Read the model definition and answer for the solid it produces. Units are mm, in the model's axes. A direction names the side the tool comes from. Give positions to 0.01 mm unless a question says otherwise; leave off trailing zeros. Write each loop counter-clockwise with the first axis right and the second up, starting at its lowest first coordinate (ties: lowest second). Pieces come first, ordered by that corner, then holes. Notation, with made-up numbers: M 40,19.25 L 64,19.25 A10 ccw 64,31.25 Z; hole C 73,48 d3. An arc over 180 degrees is marked long. Answer as CSV lines item,"result". Start each with the question number.
```python
from build123d import *

# Parameters (mm, degrees)
EXTRUDE_THIN1_DEPTH       = 100
BOSS_EXTRUDE1_START       = -10
BOSS_EXTRUDE1_DEPTH       = 10
SKETCH3_R                 = 2.25
BOSS_EXTRUDE2_DEPTH       = 5
BOSS_EXTRUDE3_DEPTH       = 10
SKETCH5_R                 = 2.25
CUT_EXTRUDE1_DEPTH        = 6
BOSS_EXTRUDE4_REACH       = 121.416
BOSS_EXTRUDE4_END_RADIUS  = 39
SKETCH10_W                = 20
SKETCH10_H                = 20
BOSS_EXTRUDE5_START       = -19.757252304
BOSS_EXTRUDE5_OUTLINE_W   = 20
BOSS_EXTRUDE5_OUTLINE_H   = 20
BOSS_EXTRUDE5_DEPTH       = 19.757252304
BOSS_EXTRUDE5_START_2     = 71.178890271
BOSS_EXTRUDE5_2_OUTLINE_W = 23
BOSS_EXTRUDE5_2_OUTLINE_H = 23
BOSS_EXTRUDE5_2_DEPTH     = 1.821109729
BOSS_EXTRUDE6_DEPTH       = 20
SKETCH12_R                = 2.5
CUT_EXTRUDE2_DEPTH        = 20


with BuildPart() as part:
    # Sketch1 → Extrude-Thin1 (new body)
    with BuildSketch(Plane.XY):
        with BuildLine():
            ThreePointArc((-35, 0), (0, -35), (35, 0))
            Line((35, 0), (39, 0))
            ThreePointArc((39, 0), (0, -39), (-39, 0))
            Line((-39, 0), (-35, 0))
        make_face()
    extrude(amount=EXTRUDE_THIN1_DEPTH)

    # Sketch2 → Boss-Extrude1 (add)
    with BuildSketch(Plane.XY.offset(100).offset(BOSS_EXTRUDE1_START)):
        with BuildLine():
            Line((0, -39), (0, -35))
            Line((0, -35), (-10, -35))
            Line((-10, -35), (-10, -37.69615365))
            ThreePointArc((-10, -37.69615365), (-5.042321274, -38.672664715), (0, -39))
        make_face()
        with BuildLine():
            Line((10, -35), (0, -35))
            Line((0, -35), (0, -39))
            ThreePointArc((0, -39), (5.042321274, -38.672664715), (10, -37.69615365))
            Line((10, -37.69615365), (10, -35))
        make_face()
        with BuildLine():
            ThreePointArc((10, -37.69615365), (5.042321274, -38.672664715), (0, -39))
            ThreePointArc((0, -39), (-5.042321274, -38.672664715), (-10, -37.69615365))
            Line((-10, -37.69615365), (-10, -43))
            Line((-10, -43), (10, -43))
            Line((10, -43), (10, -37.69615365))
        make_face()
    extrude(amount=BOSS_EXTRUDE1_DEPTH)

    # Sketch3 → Boss-Extrude2 (add)
    with BuildSketch(Plane.XY.offset(100)):
        with Locations((-5, -39)):
            Circle(SKETCH3_R)
        with Locations((5, -39)):
            Circle(SKETCH3_R)
    extrude(amount=BOSS_EXTRUDE2_DEPTH)

    # Sketch4 → Boss-Extrude3 (add)
    with BuildSketch(Plane(origin=(0, 0, 0), x_dir=(-1, 0, 0), z_dir=(0, 0, -1))):
        with BuildLine():
            Line((0, -39), (0, -35))
            Line((0, -35), (-10, -35))
            Line((-10, -35), (-10, -37.69615365))
            ThreePointArc((-10, -37.69615365), (-5.042321274, -38.672664715), (0, -39))
        make_face()
        with BuildLine():
            ThreePointArc((10, -37.69615365), (5.042321274, -38.672664715), (0, -39))
            ThreePointArc((0, -39), (-5.042321274, -38.672664715), (-10, -37.69615365))
            Line((-10, -37.69615365), (-10, -43))
            Line((-10, -43), (10, -43))
            Line((10, -43), (10, -37.69615365))
        make_face()
        with BuildLine():
            Line((10, -35), (0, -35))
            Line((0, -35), (0, -39))
            ThreePointArc((0, -39), (5.042321274, -38.672664715), (10, -37.69615365))
            Line((10, -37.69615365), (10, -35))
        make_face()
    extrude(amount=-BOSS_EXTRUDE3_DEPTH)

    # Sketch5 → Cut-Extrude1 (cut)
    with BuildSketch(Plane(origin=(0, 0, 0), x_dir=(-1, 0, 0), z_dir=(0, 0, -1))):
        with Locations(Location((-5, -39, 0), (0, 0, 180))):
            Circle(SKETCH5_R)
        with Locations(Location((5, -39, 0), (0, 0, 180))):
            Circle(SKETCH5_R)
    extrude(amount=-CUT_EXTRUDE1_DEPTH, mode=Mode.SUBTRACT)

    # Boss-Extrude4: up to this cylinder (the profile starts outside it)
    boss_extrude4_end = Plane(origin=(0, 0, 50), z_dir=(0, 0, -1)) * Cylinder(BOSS_EXTRUDE4_END_RADIUS, 321.832, mode=Mode.PRIVATE)
    # Sketch10 → Boss-Extrude4 (add, up to the surface)
    with BuildSketch(Plane(origin=(0, -51.355775573, 4.493048169), x_dir=(1, 0, 0), z_dir=(0, 0.9961946980917462, -0.08715574274765152)), mode=Mode.PRIVATE) as boss_extrude4_sk1:
        with Locations((0, -45.680780994)):
            Rectangle(SKETCH10_W, SKETCH10_H)
    boss_extrude4_tool1 = extrude(boss_extrude4_sk1.sketch, amount=BOSS_EXTRUDE4_REACH, mode=Mode.PRIVATE) - boss_extrude4_end
    add(boss_extrude4_tool1.solids().sort_by_distance((0, -47.374433, 50))[0])

    # Boss-Extrude5: read off the stored shape, not the designer's step
    # Boss-Extrude5 outline → Boss-Extrude5 (add)
    with BuildSketch(Plane(origin=(0, -51.355775573, 4.493048169), x_dir=(1, 0, 0), z_dir=(0, 0.9961946980917462, -0.08715574274765152)).offset(BOSS_EXTRUDE5_START)):
        with Locations((0, -45.680780994)):
            Rectangle(BOSS_EXTRUDE5_OUTLINE_W, BOSS_EXTRUDE5_OUTLINE_H)
    extrude(amount=BOSS_EXTRUDE5_DEPTH)

    # Boss-Extrude5 2 outline → Boss-Extrude5 2 (cut)
    with BuildSketch(Plane(origin=(0, 0, 0), x_dir=(0.9994119135527714, 0.0341374804572781, -0.0032341114416133587), z_dir=(0.034290334626361094, -0.9949568891477218, 0.09426007473315587)).offset(BOSS_EXTRUDE5_START_2)):
        with Locations((-2.5, 45.5)):
            Rectangle(BOSS_EXTRUDE5_2_OUTLINE_W, BOSS_EXTRUDE5_2_OUTLINE_H)
    extrude(amount=BOSS_EXTRUDE5_2_DEPTH, mode=Mode.SUBTRACT)

    # Sketch11 → Boss-Extrude6 (add, along a direction that is not the sketch's normal)
    with BuildSketch(Plane(origin=(10, 0, 0), x_dir=(0, 0, -1), z_dir=(1, 0, 0))):
        Polygon((-41.700202309, -67.244443924), (-40.825315674, -57.244443924), (-60.736677348, -55.358084364), (-61.611563983, -65.358084364), align=None)
    extrude(amount=BOSS_EXTRUDE6_DEPTH, dir=(0.9994118831812419, 0.03416073136677643, -0.002988676732382235))

    # Sketch12 → Cut-Extrude2 (cut)
    with BuildSketch(Plane(origin=(2.096746102, -60.838484135, 5.763707075), x_dir=(0.9994101830326217, 0.03396190638807499, -0.005086744065644943), z_dir=(-0.03429033462636107, 0.994956889147722, -0.09426007473315641))):
        with Locations(Location((17.832976273, -40.280011427, 0), (0, 0, 269.893376297))):
            Circle(SKETCH12_R)
        with Locations(Location((17.814365976, -50.280510703, 0), (0, 0, 269.893376297))):
            Circle(SKETCH12_R)
    extrude(amount=-CUT_EXTRUDE2_DEPTH, mode=Mode.SUBTRACT)


solid = part.part
```
1. Find section C-C on x = 5. Determine the outline of the cut face in (y, z).
2. Find the intervals of material crossed by line 1 (X direction, y = -39, z = 1.55); line 2 (X direction, y = -22.5, z = 59.5); line 3 (X direction, y = -15, z = 40), in increasing order. Write a range as [from, to].
3. Given pin 1 (1.6 mm diameter, centred on y = -41.5, z = 97, fed in from -X); pin 2 (12 mm diameter, centred on x = -13, y = -42, fed in from +Z); pin 3 (4 mm diameter, centred on x = 13, z = 86, fed in from -Y); pin 4 (2 mm diameter, centred on y = -41, z = 23, fed in from +X) (1 decimal), each flat-ended and moving along its own axis, determine where each tip first touches the part or whether it passes through.
4. Find section A-A on y = -24. Determine the outline of the cut face in (x, z), then the cut area to 3 significant figures.
5. Find section B-B on z = 7.5. Determine the outline of the cut face in (x, y), then the cut area to 3 significant figures.
6. Determine the mould class of faces 6 (the face through (-5, -39, 105)), 7 (the face through (-37, 0, 49)), 8 (the face through (20.91, -60.16, 58.57)) for opening direction Z: +Z half, -Z half, draft (parallel to the pull), parting line (faces both ways), or undercut.
7. Find section D-D on y = -6.5. Determine the outline of the cut face in (x, z), then the cut area to 3 significant figures.
8. For faces 1 (the face through (0, -43, 5)), 2 (the face through (10, -40, 95)), 3 (the face through (-5.29, -41.23, 2.96)), 4 (the face through (0, -43, 95)), 5 (the face through (4.71, -36.77, 102.46)), determine the directions among +Z, -Z, +X, -X, +Y, -Y from which every point of the face is accessible in a straight line to the end or side of a thin tool.
Computed:
1,outline,"M -67.42,41.72 L -38.68,39.2 L -38.68,10 L -43,10 L -43,0 L -41.25,0 L -41.25,6 L -36.75,6 L -36.75,0 L -34.64,0 L -34.64,100 L -36.75,100 L -36.75,105 L -41.25,105 L -41.25,100 L -43,100 L -43,90 L -38.68,90 L -38.68,59.28 L -65.53,61.63 Z"
2,line 1,"x = [-10, -7.25], [-2.75, 2.75], [7.25, 10]"
2,line 2,"x = [-31.86, -26.81], [26.81, 31.86]"
2,line 3,"x = [-36, -31.62], [31.62, 36]"
3,pin 1,"stops at x = -10"
3,pin 2,"stops at z = 100"
3,pin 3,"stops at y = -37.42"
3,pin 4,"passes through"
4,outline,"M -30.74,0 L -25.48,0 L -25.48,100 L -30.74,100 Z; M 25.48,0 L 30.74,0 L 30.74,100 L 25.48,100 Z"
4,area,"1,050 mm^2"
5,outline,"M -39,0 A39 ccw -10,-37.7 L -10,-43 L 10,-43 L 10,-37.7 A39 ccw 39,0 L 35,0 A35 cw -35,0 Z"
5,area,"554 mm^2"
6,face 6,"+Z half"
6,face 7,"draft"
6,face 8,"undercut"
7,outline,"M -38.45,0 L -34.39,0 L -34.39,100 L -38.45,100 Z; M 34.39,0 L 38.45,0 L 38.45,100 L 34.39,100 Z"
7,area,"813 mm^2"
8,face 1,"-Z, +X, -X, -Y"
8,face 2,"+Z, -Z, +X, -Y"
8,face 3,"-Z"
8,face 4,"+Z, +X, -X, -Y"
8,face 5,"+Z"
